```python
from build123d import *

# Parameters (mm, degrees)
BOSS_EXTRUDE1_DEPTH = 220
FILLET1_R           = 25
BOSS_EXTRUDE2_START = 3
BOSS_EXTRUDE2_DEPTH = 3
FILLET2_R           = 25


with BuildPart() as part:
    # Sketch1 → Boss-Extrude1 (new body)
    with BuildSketch(Plane(origin=(0, 0, 0), x_dir=(1, 0, 0), z_dir=(0, 1, 0))):
        Polygon((33, 107.5), (110, 107.5), (110, -107.5), (65, -107.5), (65, -112.5), (115, -112.5), (115, 112.5), (38, 112.5), (38, 178.5), (-38, 178.5), (-38, 112.5), (-115, 112.5), (-115, -112.5), (-65, -112.5), (-65, -107.5), (-110, -107.5), (-110, 107.5), (-33, 107.5), (-33, 173.5), (33, 173.5), align=None)
    extrude(amount=BOSS_EXTRUDE1_DEPTH)

    # Fillet1
    fillet1_edges = [part.edges().sort_by_distance(p)[0] for p in [
        (33, 110, -107.5),
        (-33, 110, -107.5),
        (-38, 110, -112.5),
        (38, 110, -112.5),
    ]]
    fillet(fillet1_edges, radius=FILLET1_R)

    # Sketch2 → Boss-Extrude2 (add)
    with BuildSketch(Plane(origin=(0, 220, 0), x_dir=(1, 0, 0), z_dir=(0, 1, 0)).offset(BOSS_EXTRUDE2_START)):
        with BuildLine():
            Line((-115, -112.5), (115, -112.5))
            Line((115, -112.5), (115, 112.5))
            Line((115, 112.5), (63, 112.5))
            ThreePointArc((63, 112.5), (45.32233047, 119.82233047), (38, 137.5))
            Line((38, 137.5), (38, 178.5))
            Line((38, 178.5), (-38, 178.5))
            Line((-38, 178.5), (-38, 137.5))
            ThreePointArc((-38, 137.5), (-45.32233047, 119.82233047), (-63, 112.5))
            Line((-63, 112.5), (-115, 112.5))
            Line((-115, 112.5), (-115, -112.5))
        make_face()
    extrude(amount=-BOSS_EXTRUDE2_DEPTH)

    # Fillet2
    fillet2_edges = [part.edges().sort_by_distance(p)[0] for p in [
        (110, 110, 107.5),
        (110, 110, -107.5),
        (-110, 110, -107.5),
        (-110, 110, 107.5),
        (-115, 111.5, 112.5),
        (-115, 111.5, -112.5),
        (115, 111.5, -112.5),
        (115, 111.5, 112.5),
    ]]
    fillet(fillet2_edges, radius=FILLET2_R)


solid = part.part
```
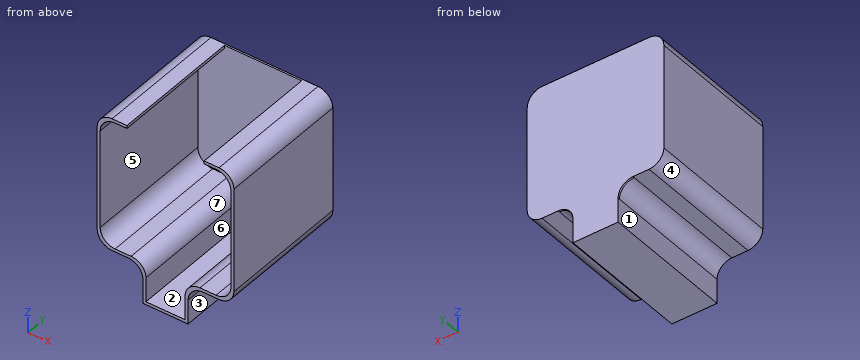
Can you work these out from the model? Positions are in its coordinate system, mm. Face numbers are marked on the shaded views. A direction names the side the tool comes from. Round coordinates to 2 decimals unless told otherwise and drop trailing zeros. Loops run counter-clockwise (first coordinate to the right, second up) from the corner with the lowest first, then second, coordinate; pieces in that order, holes last. Notation, with made-up numbers: M 2,83.5 L 42,83.5 A28 cw 42,107.5 Z; hole C 67,-35.5 d9. An arc over 180 degrees is marked long. Answer as a JSON object with one key per item and string values. Group by question number.
Q1. Imagine slicing it at D-D, the plane x = -9. Please give me the cut outline in (y, z), then the cut area to 3 significant figures.
Q2. On a 3-axis mill with a long thin cutter (end or side, diameter ignored), from which of +Z, -Z, +X, -X, +Y, -Y can I reach the whole of each face in a straight line? I mean the marked faces 1, 2 and 3. Say none if no direction works.
Q3. Will these pins go through, and if not, where does the flat tip stop? pin 1 (4 mm diameter, centred on y = 132.5, z = 109.5, fed in from +X); pin 2 (1.5 mm diameter, centred on y = 126, z = 109.5, fed in from -X); pin 3 (2 mm diameter, centred on x = 59, y = 36.5, fed in from +Z).
Q4. Please list where these lines run through material, in increasing order: L1, parallel to Z at x = 78.5, y = 176; L2, parallel to X at y = 147.5, z = 26; L3, parallel to X at y = 84, z = -161.5.
Q5. Imagine slicing it at C-C, the plane x = -80. Please give me the cut outline in (y, z), then the cut area to 4 significant figures.
Q6. Imagine slicing it at A-A, the plane z = -23. Please give me the cut outline in (x, y), then the cut area to 3 significant figures.
Q7. We'd pull the mould along Z, two halves only. Please class the marked faces 4, 5, 6 and 7: +Z half, -Z half, draft (parallel to the pull), parting line (faces both ways), or undercut.
Findings:
{
 "1": {"outline": "M 0,-178.5 L 223,-178.5 L 223,112.5 L 220,112.5 L 220,-173.5 L 0,-173.5 Z", "area": "1,970 mm2"},
 "2": {"face 1": "-Z, -X, +Y, -Y", "face 2": "+Z, -Y", "face 3": "-Z, +X, +Y, -Y"},
 "3": {"pin 1": "stops at x = 105", "pin 2": "stops at x = -103.17", "pin 3": "stops at z = -107.5"},
 "4": {"L1": "z = -112.5 to -107.5, 107.5 to 112.5", "L2": "x = -115 to -110, 110 to 115", "L3": "x = -38 to -33, 33 to 38"},
 "5": {"outline": "M 0,-112.5 L 223,-112.5 L 223,112.5 L 0,112.5 L 0,107.5 L 220,107.5 L 220,-107.5 L 0,-107.5 Z", "area": "2,875 mm2"},
 "6": {"outline": "M -115,0 L -110,0 L -110,220 L 110,220 L 110,0 L 115,0 L 115,223 L -115,223 Z", "area": "2,890 mm2"},
 "7": {"face 4": "-Z half", "face 5": "undercut", "face 6": "draft", "face 7": "+Z half"}
}
